```python
from build123d import *

# Parameters (mm, degrees)
BOSS_EXTRUDE1_DEPTH = 5
SKETCH2_R           = 7.5
BOSS_EXTRUDE2_DEPTH = 87.988181024
SKETCH3_R           = 3
CUT_EXTRUDE1_DEPTH  = 87.988181024
CUT_EXTRUDE2_DEPTH  = 5
BOSS_EXTRUDE3_DEPTH = 6.928203
CUT_EXTRUDE3_START  = -0.5
SKETCH10_W          = 96.059977794
SKETCH10_H          = 5
CUT_EXTRUDE3_DEPTH  = 10.5
BOSS_EXTRUDE4_START = 1
SKETCH11_R          = 1.5
BOSS_EXTRUDE4_DEPTH = 5
FILLET1_R           = 1
FILLET2_R           = 3


with BuildPart() as part:
    # Sketch1 → Boss-Extrude1 (new body)
    with BuildSketch(Plane(origin=(0, 0, 0), x_dir=(1, 0, 0), z_dir=(0, 1, 0))):
        Polygon((0, 87.988181024), (0, 0), (-76.2, 43.994090512), (-91.2, 69.974852626), (-15, 113.968943138), align=None)
    extrude(amount=BOSS_EXTRUDE1_DEPTH)

    # Sketch2 → Boss-Extrude2 (add)
    with BuildSketch(Plane(origin=(-38.1, 0, 21.997045256), x_dir=(0.49999999999999967, 0, 0.8660254037844388), z_dir=(-0.8660254037844388, 0, 0.49999999999999967))):
        with Locations((-99.128932188, 2.5)):
            Circle(SKETCH2_R)
    extrude(amount=-BOSS_EXTRUDE2_DEPTH)

    # Sketch3 → Cut-Extrude1 (cut)
    with BuildSketch(Plane(origin=(-38.1, 0, 21.997045256), x_dir=(0.49999999999999967, 0, 0.8660254037844388), z_dir=(-0.8660254037844388, 0, 0.49999999999999967))):
        with Locations((-99.128932188, 2.5)):
            Circle(SKETCH3_R)
    extrude(amount=-CUT_EXTRUDE1_DEPTH, mode=Mode.SUBTRACT)

    # Sketch5 → Cut-Extrude2 (cut)
    with BuildSketch(Plane(origin=(0, 5, 0), x_dir=(1, 0, 0), z_dir=(0, 1, 0))):
        Polygon((-6, 3.464101615), (0, 6.92820323), (0, 0), align=None)
    extrude(amount=-CUT_EXTRUDE2_DEPTH, mode=Mode.SUBTRACT)

    # Sketch7 → Boss-Extrude3 (add)
    with BuildSketch(Plane(origin=(-3, 0, 1.732050808), x_dir=(0, 1, 0), z_dir=(0.8660254037844383, 0, -0.5000000000000006))):
        Polygon((0.833333333, -4), (0, -6), (1.666666667, -6), align=None)
        Polygon((2.5, -4), (1.666666667, -6), (3.333333333, -6), align=None)
        Polygon((4.166666667, -4), (3.333333333, -6), (5, -6), align=None)
    extrude(amount=BOSS_EXTRUDE3_DEPTH)

    # Sketch10 → Cut-Extrude3 (cut)
    with BuildSketch(Plane(origin=(0, 0, 0), x_dir=(0.8660254037844386, 0, 0.5000000000000001), z_dir=(-0.5000000000000001, 0, 0.8660254037844386)).offset(CUT_EXTRUDE3_START)):
        with Locations((-44.958192127, 2.5)):
            Rectangle(SKETCH10_W, SKETCH10_H)
    cut_extrude3 = extrude(amount=CUT_EXTRUDE3_DEPTH, mode=Mode.SUBTRACT)

    # Mirror1: Cut-Extrude3 across plane
    add(cut_extrude3.mirror(Plane(origin=(0, 0, 0), x_dir=(0.4999999999999997, 0, 0.8660254037844387), z_dir=(0.8660254037844387, 0, -0.49999999999999983))), mode=Mode.SUBTRACT)

    # Sketch11 → Boss-Extrude4 (add)
    with BuildSketch(Plane(origin=(0, 0, 0), x_dir=(-0.49999999999999983, 0, -0.8660254037844387), z_dir=(0.8660254037844387, 0, -0.49999999999999983)).offset(BOSS_EXTRUDE4_START)):
        with BuildLine():
            Line((53.800614721, 12.707564932), (51, 5))
            Line((51, 5), (66, 5))
            Line((66, 5), (63.199385279, 12.707564932))
            ThreePointArc((63.199385279, 12.707564932), (58.5, 16), (53.800614721, 12.707564932))
        make_face()
        with Locations(Location((58.5, 11, 0), (0, 0, 180))):
            Circle(SKETCH11_R, mode=Mode.SUBTRACT)
    boss_extrude4 = extrude(amount=BOSS_EXTRUDE4_DEPTH)

    # Mirror2: Boss-Extrude4 across plane
    add(boss_extrude4.mirror(Plane(origin=(0, 0, 0), x_dir=(0.4999999999999997, 0, 0.8660254037844387), z_dir=(0.8660254037844387, 0, -0.49999999999999983))))

    # Fillet1
    fillet1_edges = [part.edges().sort_by_distance(p)[0] for p in [
        (-24.053847577, 5, -53.662486121),
        (-28.383974596, 5, -51.162486121),
        (-22.468911087, 5, -45.917295593),
        (-29.968911087, 5, -58.90767665),
        (-34.446152423, 5, -47.662486121),
        (-36.031088913, 5, -55.40767665),
        (-28.531088913, 5, -42.417295593),
        (-30.116025404, 5, -50.162486121),
    ]]
    fillet(fillet1_edges, radius=FILLET1_R - 0.0001)  # a hair under: the kernel refuses the full size

    # Fillet2
    fillet2_edges = [part.edges().sort_by_distance(p)[0] for p in [
        (-46.028932188, 0, -79.724449168),
        (-46.028932188, 5, -79.724449168),
    ]]
    fillet(fillet2_edges, radius=FILLET2_R)


solid = part.part
```
Can you work these out from the model? Positions are in its coordinate system, mm. A direction names the side the tool comes from. Coordinates: 2 decimals unless noted, no trailing zeros. Loops run counter-clockwise (first coordinate to the right, second up) from the corner with the lowest first, then second, coordinate; pieces in that order, holes last.
1) For pin 1 (12 mm diameter, centred on x = -34, z = -34, fed in from +Y); pin 2 (10 mm diameter, centred on x = -22, y = 3, fed in from -Z); pin 3 (4 mm diameter, centred on x = -15, y = -0.5, fed in from +Z), each with a flat end and sliding along its axis, tell me the tip position at first contact or that it passes through.
2) Thinking about a two-plate mould opening in Z: for faces 4 (the flat face through (-28.334, 8.848, -51.076)), 5 (the cylindrical face through (-26.3, 16, -52.5)), 6 (the flat face through (-2.54, 4.59, -4.32)), which applies, pulls with the +Z half, pulls with the -Z half, needs draft (parallel to the pull), parting line crosses it, or undercut?
3) I need wall thicknesses on probe 1 along Y at (x, z) = (-6, -23); probe 2 along Z at (x, y) = (-75.5, 3.5); probe 3 along Z at (x, y) = (-82, 3.5). Which ranges of each line are inside material? Lowest first, please.
4) Imagine slicing it at A-A on y = -3.5. List the corners of the cut face in (x, z) for me.
5) Which directions (+Z, -Z, +X, -X, +Y, -Y) give clear straight access to the entire face, cutting with the end or side of a thin tool? Please do faces 1 (the flat face through (-32, 0, -53)), 2 (the flat face through (-35.249, 9.134, -54.125)), 3 (the flat face through (-24.004, 8.848, -53.576)).
6) Imagine slicing it at B-B on z = -15. List the corners of the cut face in (x, y) for me.
Completed:
1. pin 1: stops at y = 5
1. pin 2: stops at z = -113.3
1. pin 3: stops at z = -8.12
2. face 4: undercut
2. face 5: parting line crosses it
2. face 6: pulls with the +Z half
3. probe 1: y = 0 to 5
3. probe 2: z = -79.46 to -74.14, -67.61 to -44.17
3. probe 3: z = -75.7 to -70.39, -63.86 to -54.04
4. outline: (-89.91, -67.75) - (-13.71, -111.74) - (-9.21, -103.95) - (-85.41, -59.95) - close
5. face 1: +Z, +X, -Y
5. face 2: -X, +Y
5. face 3: +X, +Y
6. outline: (-24.98, 0) - (-0.5, 0) - (-0.5, 5) - (-24.98, 5) - close
